from build123d import *

# Parameters (mm, degrees)
SKETCH2_W          = 0.5
SKETCH2_H          = 4.582575694
CUT_EXTRUDE1_DEPTH = 16.667163113
SKETCH3_W          = 0.5
SKETCH3_H          = 0.5


with BuildPart() as part:
    # Sketch1 → Revolve1 (revolve)
    with BuildSketch(Plane(origin=(0, 0, 0), x_dir=(1, 0, 0), z_dir=(0, 1, 0))):
        with BuildLine():
            Line((0, 0), (0, 13.6))
            ThreePointArc((0, 13.6), (3.535533906, 12.135533906), (5, 8.6))
            Line((5, 8.6), (5, 2))
            Line((5, 2), (5.5, 2))
            Line((5.5, 2), (5.5, 0))
            Line((5.5, 0), (0, 0))
        make_face()
    revolve(axis=Axis((0, 0, 0), (0, 0, -1)))

    # Sketch2 → Cut-Extrude1 (cut, through all)
    with BuildSketch(Plane.XY):
        with Locations((5.25, 0)):
            Rectangle(SKETCH2_W, SKETCH2_H)
    extrude(amount=-CUT_EXTRUDE1_DEPTH, mode=Mode.SUBTRACT)

    # Sweep1: sweep along a path in Sketch4
    with BuildLine(Plane(origin=(1.27, 0, 0), x_dir=(0, 0, -1), z_dir=(1, 0, 0))) as sweep1_path:
        Line((0, 0), (-0.4, 0))
        ThreePointArc((-0.4, 0), (-1.107106781, -0.292893219), (-1.4, -1))
        Line((-1.4, -1), (-1.4, -8))
    # Sketch3 → Sweep1 (sweep)
    with BuildSketch(Plane.XY):
        with Locations((-1.27, 0)):
            Rectangle(SKETCH3_W, SKETCH3_H)
        with Locations((1.27, 0)):
            Rectangle(SKETCH3_W, SKETCH3_H)
    sweep(path=sweep1_path.line)


solid = part.part
Part model, mm, in its own coordinate system. A direction names the side the tool comes from. Coordinates: 2 decimals unless noted, no trailing zeros. Loops run counter-clockwise (first coordinate to the right, second up) from the corner with the lowest first, then second, coordinate; pieces in that order, holes last. Notation, with made-up numbers: (9.5, 70.25) -> (30.5, 70.25) arc R11 cw to (30.5, 89.25) -> close; hole circle Ø7 at (22.25, 56.25). An arc over 180 degrees is marked (long way). Use a Markdown table: item, result. Add a question column.
Item 1: Which spindle directions (+Z, -Z, +X, -X, +Y, -Y) get a long thin tool onto all of the face, cutting with end or side? Do faces 4 (the cylindrical face through (-1.08, 4.88, -5.25)), 5 (the flat face through (1.52, -3.6, 1.3)), 6 (the flat face through (-1.52, -2.9, 1.4)). Say none if no direction does.
Item 2: Band-saw the part on D-D on y = -1.75. Write the cut outline in (x, z).
Item 3: Band-saw the part on C-C on z = -4. Write the cut outline in (x, y), plus the area to 3 significant figures.
Item 4: Band-saw the part on A-A on y = -4.5. Write the cut outline in (x, z).
Item 5: Probe probe 1 along Z at (x, y) = (4.25, 3); probe 2 along X at (y, z) = (-0.5, -1.75); probe 3 along Y at (x, z) = (-4, -0.5). List the from-to ranges inside material, lowest first.
Item 6: Flat gauge pins, fed straight in: P1, Ø8, axis at y = -1.5, z = -9.5, coming from the -X side; P2, Ø2, axis at x = -4, y = 0, coming from the -Z side; P3, Ø1.5, axis at x = -2, y = 0.5, coming from the +Z side. Where does each tip first touch, or does it go through?
Item 7: Pull direction X, two halves, no side cores. Call faces 1 (the flat face through (1.02, -2.9, 1.4)), 2 (the cylindrical face through (-1.274, -0.106, 1.274)), 3 (the cylindrical face through (-5.496, -0.209, -0.986)): +X half, -X half, draft (parallel to the pull), parting line (faces both ways), or undercut.
Item 8: Band-saw the part on B-B on x = 0. Write the cut outline in (y, z).
Geometry says:
| question | item | result |
|---|---|---|
| 1 | face 4 | -Z |
| 1 | face 5 | +Z, +X, +Y, -Y |
| 1 | face 6 | +Z, -X, +Y, -Y |
| 2 | outline | (-5.21, -2) -> (-4.68, -2) -> (-4.68, -8.6) arc R4.68 ccw to (4.68, -8.6) -> (4.68, -2) -> (5, -2) -> (5, 0) -> (-5.21, 0) -> close; (-1.52, 1.15) -> (-1.02, 1.15) -> (-1.02, 1.65) -> (-1.52, 1.65) -> close; (1.02, 1.15) -> (1.52, 1.15) -> (1.52, 1.65) -> (1.02, 1.65) -> close |
| 3 | outline | circle Ø10 at (0, 0) |
| 3 | area | 78.5 mm² |
| 4 | outline | (-3.16, -2) -> (-2.18, -2) -> (-2.18, -8.6) arc R2.18 ccw to (2.18, -8.6) -> (2.18, -2) -> (3.16, -2) -> (3.16, 0) -> (-3.16, 0) -> close; (-1.52, 1.15) -> (-1.02, 1.15) -> (-1.02, 1.65) -> (-1.52, 1.65) -> close; (1.02, 1.15) -> (1.52, 1.15) -> (1.52, 1.65) -> (1.02, 1.65) -> close |
| 5 | probe 1 | -2 to 0 |
| 5 | probe 2 | -5.48 to 5 |
| 5 | probe 3 | -3.77 to 3.77 |
| 6 | P1 | x = -5 |
| 6 | P2 | z = -12.6 |
| 6 | P3 | z = 1.24 |
| 7 | face 1 | undercut |
| 7 | face 2 | draft |
| 7 | face 3 | parting line |
| 8 | outline | (-5.5, -2) -> (-5, -2) -> (-5, -8.6) arc R5 ccw to (5, -8.6) -> (5, -2) -> (5.5, -2) -> (5.5, 0) -> (-5.5, 0) -> close |
